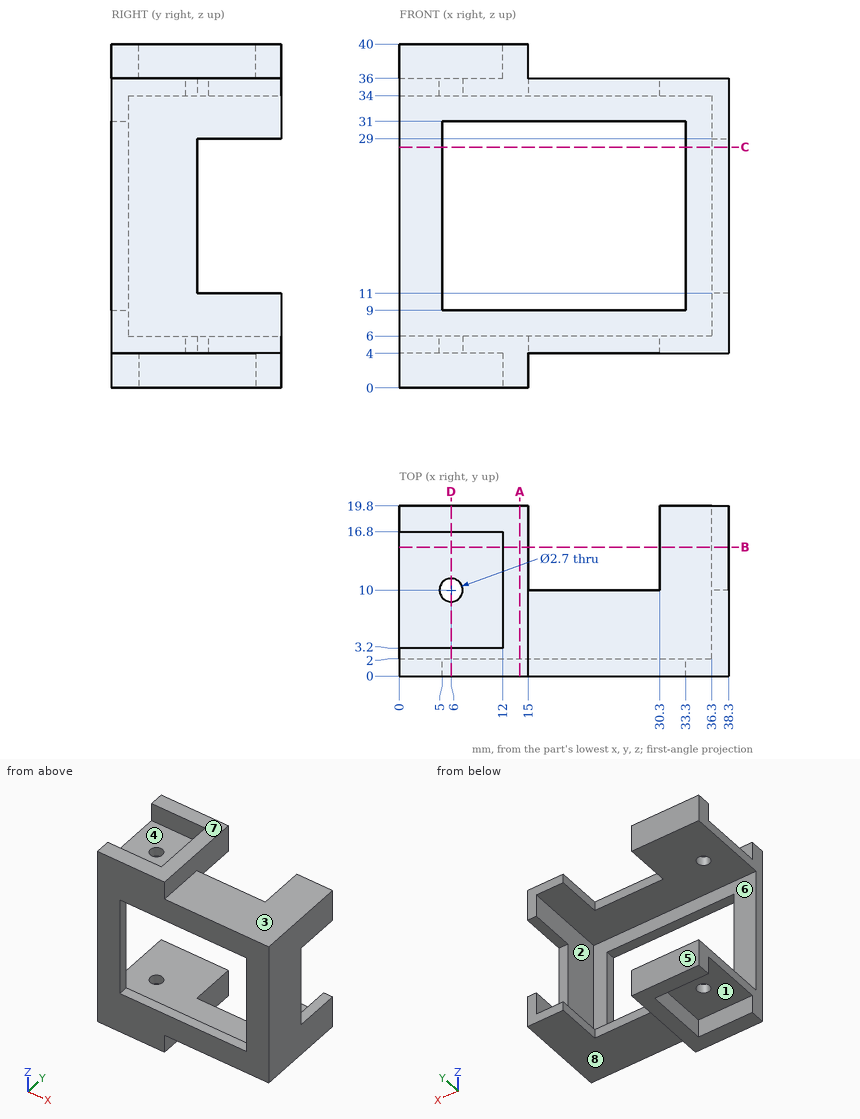
Geometry check sheet. Reference: drawing and pictorial views, mm from the part's lowest x, y, z. A direction names the side the tool comes from. Round coordinates to 2 decimals unless told otherwise and drop trailing zeros. Order: outer loops, then holes, each group sorted by start corner. A loop starts at its lowest first (then second) coordinate and runs counter-clockwise, first axis right, second up. Notation, with made-up numbers: (73.25, 41) - (115.25, 41) arc R21 cw to (115.25, 61) - close; hole circle Ø3 at (-23, 65.5). An arc over 180 degrees is marked (long way). Use a Markdown table: item, result. Add a question column.
1) Section check C-C (z = 28). Record the cut outline in (x, y), then the cut area to 3 significant figures.
2) Section check B-B (y = 15). Record the cut outline in (x, z), then the cut area to 3 significant figures.
3) Set-up check for the marked faces 1, 2, 3 and 4: record each of +Z, -Z, +X, -X, +Y, -Y from which the full face is reachable in a straight line by a thin tool's end or side.
4) Mould release check, pull along Z, two halves, no side actions. Record for the marked faces 5, 6, 7 and 8: released by +Z, released by -Z, zero draft, split by the parting line, or undercut.
5) Section check D-D (x = 6). Record the cut outline in (y, z), then the cut area to 3 significant figures.
6) Gauge pin test, flat ends, axial feed: P1, Ø1, axis at y = 14, z = 5.5, coming from the -X side; P2, Ø3, axis at x = 18.5, y = 4, coming from the -Z side; P3, Ø1, axis at x = 37, y = 14, coming from the +Z side; P4, Ø2.5, axis at x = 6, y = 10, coming from the +Z side. Record the tip position at first contact, or that the pin passes through.
7) Section check A-A (x = 14). Record the cut outline in (y, z).
8) Thickness scan on line 1 along Z through (x, y) = (32, 15.75); line 2 along Y through (x, z) = (6, 5.65); line 3 along Z through (x, y) = (36.5, 19.25). Record the ranges inside material, lowest first.
Established:
| question | item | result |
|---|---|---|
| 1 | outline | (0, 0) - (5, 0) - (5, 2) - (0, 2) - close; (33.3, 0) - (38.3, 0) - (38.3, 10) - (36.3, 10) - (36.3, 2) - (33.3, 2) - close |
| 1 | area | 36.0 mm2 |
| 2 | outline | (0, 4) - (12, 4) - (12, 0) - (15, 0) - (15, 6) - (0, 6) - close; (0, 34) - (15, 34) - (15, 40) - (12, 40) - (12, 36) - (0, 36) - close; (30.3, 4) - (38.3, 4) - (38.3, 11) - (36.3, 11) - (36.3, 6) - (30.3, 6) - close; (30.3, 34) - (36.3, 34) - (36.3, 29) - (38.3, 29) - (38.3, 36) - (30.3, 36) - close |
| 2 | area | 136 mm2 |
| 3 | face 1 | -Z, -X |
| 3 | face 2 | -X, +Y |
| 3 | face 3 | +Z, +X, +Y, -Y |
| 3 | face 4 | +Z, -X |
| 4 | face 5 | zero draft |
| 4 | face 6 | undercut |
| 4 | face 7 | released by +Z |
| 4 | face 8 | released by -Z |
| 5 | outline | (0, 0) - (3.2, 0) - (3.2, 4) - (8.65, 4) - (8.65, 6) - (2, 6) - (2, 9) - (0, 9) - close; (0, 31) - (2, 31) - (2, 34) - (8.65, 34) - (8.65, 36) - (3.2, 36) - (3.2, 40) - (0, 40) - close; (11.35, 4) - (16.8, 4) - (16.8, 0) - (19.8, 0) - (19.8, 6) - (11.35, 6) - close; (11.35, 34) - (19.8, 34) - (19.8, 40) - (16.8, 40) - (16.8, 36) - (11.35, 36) - close |
| 5 | area | 130 mm2 |
| 6 | P1 | x = 0 |
| 6 | P2 | z = 4 |
| 6 | P3 | z = 36 |
| 6 | P4 | through |
| 7 | outline | (0, 0) - (19.8, 0) - (19.8, 6) - (2, 6) - (2, 9) - (0, 9) - close; (0, 31) - (2, 31) - (2, 34) - (19.8, 34) - (19.8, 40) - (0, 40) - close |
| 8 | line 1 | 4 to 6, 34 to 36 |
| 8 | line 2 | 0 to 8.65, 11.35 to 19.8 |
| 8 | line 3 | 4 to 11, 29 to 36 |
